Here's how the part is built. I have some questions about the finished solid (model axes, mm). Face numbers are marked on the shaded views. A direction names the side the tool comes from. Give positions to 0.01 mm unless a question says otherwise; leave off trailing zeros. Write each loop counter-clockwise with the first axis right and the second up, starting at its lowest first coordinate (ties: lowest second). Pieces come first, ordered by that corner, then holes. Notation, with made-up numbers: (-39, 89.25) -> (18, 89.25) arc R30 cw to (18, 117.25) -> close; hole circle Ø5 at (17, -30.75). An arc over 180 degrees is marked (long way). Use CSV: the item, a comma, the result in double quotes. Start each with the question number.
(1) If we mould it in two halves opening along Y, with no side actions, what happens to the marked faces 1, 2 and 3? For each: pulls with the +Y half, pulls with the -Y half, needs draft (parallel to the pull), parting line crosses it, or undercut.
(2) Which directions (+Z, -Z, +X, -X, +Y, -Y) give clear straight access to the entire face, cutting with the end or side of a thin tool? Please do the marked faces 4, 5 and 6.
(3) Suppose I cut it at A-A on z = -22.5. List the corners of the cut face in (x, y) for me.
(4) For pin 1 Ø4 at (x, z) = (-25.5, 39.5) entering from -Y; pin 2 Ø18 at (y, z) = (0, 41) entering from +X; pin 3 Ø22.5 at (x, z) = (17, -13.5) entering from +Y; pin 4 Ø10 at (x, z) = (-33.5, -9.5) entering from -Y, each with a flat end and sliding along its axis, tell me the tip position at first contact or that it passes through.
(5) Suppose I cut it at C-C on y = 122. List the corners of the cut face in (x, z) for me, plus the area to 3 significant figures.
(6) Suppose I cut it at D-D on y = 0. Give the number of separate pieces and of enclosed holes in the cut face, plus the area to 3 significant figures.
(7) I need wall thicknesses on L1, parallel to Z at x = 0, y = 93; L2, parallel to X at y = 33, z = -20; L3, parallel to Z at x = -31.5, y = -17. Which ranges of each line are inside material? Lowest first, please. Write a range as [from, to].
(8) Suppose I cut it at B-B on x = -125. List the corners of the cut face in (y, z) for me.
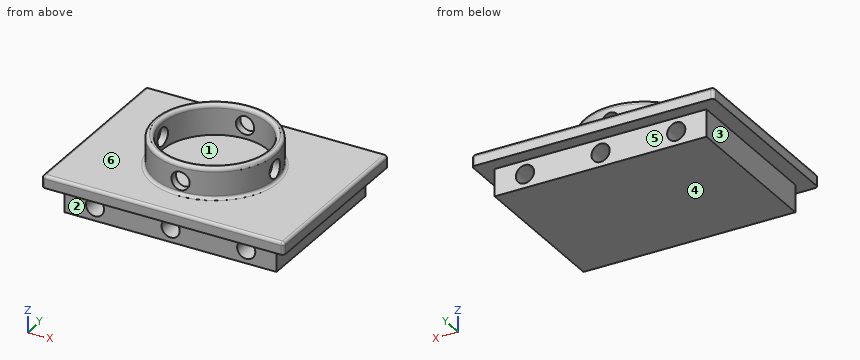
from build123d import *

# Parameters (mm, degrees)
F0_W      = 400
F0_H      = 300
F1_DEPTH  = 20
F2_R      = 100
F2_R_2    = 87.5
F3_DEPTH  = 50
F4_R      = 6
F6_R      = 15
F7_DEPTH  = 200
F9_R      = 15
F10_DEPTH = 200
F11_W     = 350
F11_H     = 255
F12_DEPTH = 45
F13_R     = 15
F14_DEPTH = 255
F15_DEPTH = 256
F16_R     = 5


with BuildPart() as f1:
    # F0 (on Top) → F1 (new body)
    with BuildSketch(Plane.XY):
        Rectangle(F0_W, F0_H)
    extrude(amount=F1_DEPTH)

    # F2 (on face) → F3 (join)
    with BuildSketch(Plane.XY.offset(20)):
        Circle(F2_R)
        Circle(F2_R_2, mode=Mode.SUBTRACT)
    extrude(amount=F3_DEPTH)

    # F4
    f4_edges = [f1.edges().sort_by_distance(p)[0] for p in [
        (-100, 0, 70),
        (-87.5, 0, 70),
    ]]
    fillet(f4_edges, radius=F4_R)

    # F6 (on offset) → F7 (cut)
    with BuildSketch(Plane.XZ.offset(100)):
        with Locations((0, 42)):
            Circle(F6_R)
    extrude(amount=-F7_DEPTH, mode=Mode.SUBTRACT)

    # F9 (on offset) → F10 (cut)
    with BuildSketch(Plane.YZ.offset(-100)):
        with Locations((0, 41)):
            Circle(F9_R)
    extrude(amount=F10_DEPTH, mode=Mode.SUBTRACT)

    # F11 (on face) → F12 (join)
    with BuildSketch(Plane(origin=(0, 0, 0), x_dir=(1, 0, 0), z_dir=(0, 0, -1))):
        Rectangle(F11_W, F11_H)
    extrude(amount=F12_DEPTH)

    # F13 (on face) → F14 (cut)
    with BuildSketch(Plane.XZ.offset(127.5)):
        with Locations((-125, -22.5)):
            Circle(F13_R)
    extrude(amount=-F14_DEPTH, mode=Mode.SUBTRACT)

    # F13 (on face) → F15 (cut)
    with BuildSketch(Plane.XZ.offset(127.5)):
        with Locations((-125, -22.5)):
            Circle(F13_R)
        with Locations((125, -22.5)):
            Circle(F13_R)
        with Locations((0, -22.5)):
            Circle(F13_R)
    extrude(amount=-F15_DEPTH, mode=Mode.SUBTRACT)

    # F16
    f16_edges = [f1.edges().sort_by_distance(p)[0] for p in [
        (0, -150, 20),
        (-200, 0, 20),
        (200, 0, 20),
        (0, 150, 20),
        (-100, 0, 20),
        (-200, -150, 10),
        (200, -150, 10),
        (200, 150, 10),
        (-200, 150, 10),
    ]]
    fillet(f16_edges, radius=F16_R)


solid = f1.part
Geometry says:
1,face 1,"undercut"
1,face 2,"pulls with the -Y half"
1,face 3,"needs draft"
2,face 4,"-Z, +X, -X, +Y, -Y"
2,face 5,"-Z, +X, -X, +Y"
2,face 6,"+Z"
3,outline,"(-175, -127.5) -> (-140, -127.5) -> (-140, 127.5) -> (-175, 127.5) -> close; (-110, -127.5) -> (-15, -127.5) -> (-15, 127.5) -> (-110, 127.5) -> close; (15, -127.5) -> (110, -127.5) -> (110, 127.5) -> (15, 127.5) -> close; (140, -127.5) -> (175, -127.5) -> (175, 127.5) -> (140, 127.5) -> close"
4,pin 1,"y = -97.2"
4,pin 2,"through"
4,pin 3,"y = 127.5"
4,pin 4,"y = -127.5"
5,outline,"(-200, 0) -> (-175, 0) -> (-175, -45) -> (175, -45) -> (175, 0) -> (200, 0) -> (200, 15) arc R5 ccw to (195, 20) -> (-195, 20) arc R5 ccw to (-200, 15) -> close; hole circle Ø30 at (-125, -22.5); hole circle Ø30 at (0, -22.5); hole circle Ø30 at (125, -22.5)"
5,area,"21,600 mm²"
6,separate pieces,"3"
6,enclosed holes,"3"
6,area,"22,100 mm²"
7,L1,"[-45, -37.5], [-7.5, 27], [57, 69.98]"
7,L2,"[-175, -139.79], [-110.21, -14.79], [14.79, 110.21], [139.79, 175]"
7,L3,"[-45, 20]"
8,outline,"(-150, 0) -> (-127.5, 0) -> (-127.5, -7.5) -> (127.5, -7.5) -> (127.5, 0) -> (150, 0) -> (150, 15) arc R5 ccw to (145, 20) -> (-145, 20) arc R5 ccw to (-150, 15) -> close; (-127.5, -45) -> (127.5, -45) -> (127.5, -37.5) -> (-127.5, -37.5) -> close"
